Source: CAD feature listing. Evaluate the final solid. Frame: model axes, mm. A direction names the side the tool comes from. Coordinates: 2 decimals unless noted, no trailing zeros. Loops run counter-clockwise (first coordinate to the right, second up) from the corner with the lowest first, then second, coordinate; pieces in that order, holes last. Notation, with made-up numbers: (14, -16.5) -> (30, -16.5) arc R30 ccw to (30, 22.5) -> close; hole circle Ø4 at (-3, -26). An arc over 180 degrees is marked (long way). Answer as a JSON object with one key per item and string values. Group by question number.
from build123d import *

# Parameters (mm, degrees)
SKETCH1_R          = 16.66875
EXTRUDE1_DEPTH     = 50.8
SKETCH2_R          = 6.35
CUT_EXTRUDE1_DEPTH = 25.4
SKETCH3_R          = 7.9375
CUT_EXTRUDE2_DEPTH = 25.4


with BuildPart() as part:
    # Sketch1 → Extrude1 (new body)
    with BuildSketch(Plane(origin=(0, 0, 0), x_dir=(0, 0, -1), z_dir=(1, 0, 0))):
        Circle(SKETCH1_R)
    extrude(amount=EXTRUDE1_DEPTH)

    # Sketch2 → Cut-Extrude1 (cut)
    with BuildSketch(Plane(origin=(50.8, 0, 0), x_dir=(0, 0, -1), z_dir=(1, 0, 0))):
        Circle(SKETCH2_R)
    extrude(amount=-CUT_EXTRUDE1_DEPTH, mode=Mode.SUBTRACT)

    # Sketch3 → Cut-Extrude2 (cut)
    with BuildSketch(Plane.ZY):
        Circle(SKETCH3_R)
    extrude(amount=-CUT_EXTRUDE2_DEPTH, mode=Mode.SUBTRACT)


solid = part.part
1. Ray query, L1, parallel to Y at x = 32.25, z = 0; L2, parallel to X at y = 7, z = 0; L3, parallel to Y at x = 19.5, z = 0. Return the intervals inside material, ascending.
2. Section query C-C on x = 45.5. Return loops of the section in (y, z), then the cut area to 3 significant figures.
3. Section query A-A on z = 0. Return loops of the section in (x, y).
4. Mould query, pull axis Z, two halves, no side actions, for faces 3 (the face through (25, 5, -15.9)), 4 (the face through (12.52, -7.75, -1.72)), 5 (the face through (50.8, -7, 0)), 6 (the face through (38.28, -6.2, 1.38)). Classes: pulls with the +Z half, pulls with the -Z half, needs draft (parallel to the pull), parting line crosses it, or undercut.
5. Reachability of faces 1 (the face through (0, 3.9, -7.2)), 2 (the face through (25.4, 7, 0)) from +Z, -Z, +X, -X, +Y, -Y: full face, straight path, thin tool, end or side. Return the list, or none.
6. Section query D-D on z = -11.5. Return loops of the section in (x, y), then the cut area to 3 significant figures.
7. Pin query (flat end, axial travel): pin 1 Ø12.5 at (y, z) = (0, 0) entering from -X; pin 2 Ø2 at (x, y) = (9, -8.5) entering from -Z; pin 3 Ø2 at (x, y) = (35, 13) entering from +Z; pin 4 Ø12 at (x, z) = (14, 9.5) entering from +Y. Return the tip coordinate at first contact, or that it passes through.
Solved:
{
 "1": {"L1": "-16.67 to -6.35, 6.35 to 16.67", "L2": "25.4 to 50.8", "L3": "-16.67 to -7.94, 7.94 to 16.67"},
 "2": {"outline": "circle Ø33.34 at (0, 0); hole circle Ø12.7 at (0, 0)", "area": "746 mm^2"},
 "3": {"outline": "(0, -16.67) -> (50.8, -16.67) -> (50.8, -6.35) -> (25.4, -6.35) -> (25.4, -7.94) -> (0, -7.94) -> close; (0, 7.94) -> (25.4, 7.94) -> (25.4, 6.35) -> (50.8, 6.35) -> (50.8, 16.67) -> (0, 16.67) -> close"},
 "4": {"face 3": "parting line crosses it", "face 4": "undercut", "face 5": "needs draft", "face 6": "undercut"},
 "5": {"face 1": "+Z, -Z, -X, +Y, -Y", "face 2": "-X"},
 "6": {"outline": "(0, -12.07) -> (50.8, -12.07) -> (50.8, 12.07) -> (0, 12.07) -> close", "area": "1,230 mm^2"},
 "7": {"pin 1": "through", "pin 2": "z = -14.89", "pin 3": "z = 11.57", "pin 4": "y = 16.3"}
}
